from build123d import *

# Parameters (mm, degrees)
SKETCH1_R           = 4
BOSS_EXTRUDE1_DEPTH = 54
SKETCH2_R           = 10
BOSS_EXTRUDE2_DEPTH = 12
SKETCH3_W           = 15
SKETCH3_H           = 30
CUT_EXTRUDE1_DEPTH  = 150
FILLET1_R           = 1


with BuildPart() as part:
    # Sketch1 → Boss-Extrude1 (new body)
    with BuildSketch(Plane.XY):
        with BuildLine():
            Line((0, 75), (0, 20))
            Line((0, 20), (-80, 20))
            ThreePointArc((-80, 20), (-100, 0), (-80, -20))
            Line((-80, -20), (0, -20))
            Line((0, -20), (0, -75))
            Line((0, -75), (15, -75))
            Line((15, -75), (15, 75))
            Line((15, 75), (0, 75))
        make_face()
        with Locations((7.5, 60)):
            Circle(SKETCH1_R, mode=Mode.SUBTRACT)
        with Locations((7.5, -60)):
            Circle(SKETCH1_R, mode=Mode.SUBTRACT)
    extrude(amount=BOSS_EXTRUDE1_DEPTH)

    # Sketch2 → Boss-Extrude2 (add)
    with BuildSketch(Plane(origin=(0, 0, 0), x_dir=(-1, 0, 0), z_dir=(0, 0, -1))):
        with Locations((80, 0)):
            Circle(SKETCH2_R)
    boss_extrude2 = extrude(amount=BOSS_EXTRUDE2_DEPTH)

    # Mirror1: Boss-Extrude2 across plane
    add(boss_extrude2.mirror(Plane.XY.offset(27)))

    # Sketch3 → Cut-Extrude1 (cut)
    with BuildSketch(Plane(origin=(0, 75, 0), x_dir=(1, 0, 0), z_dir=(0, 1, 0))):
        with Locations((7.5, -27)):
            Rectangle(SKETCH3_W, SKETCH3_H)
    extrude(amount=-CUT_EXTRUDE1_DEPTH, mode=Mode.SUBTRACT)

    # Fillet1
    fillet1_edges = [part.edges().sort_by_distance(p)[0] for p in [
        (0, -47.5, 0),
        (-40, -20, 0),
        (-100, 0, 0),
        (0, -47.5, 54),
        (0, 47.5, 54),
        (-40, 20, 54),
        (-100, 0, 54),
        (0, -47.5, 42),
        (0, 47.5, 42),
        (0, -47.5, 12),
        (0, 47.5, 12),
        (-40, 20, 0),
        (-40, -20, 54),
        (0, 47.5, 0),
    ]]
    fillet(fillet1_edges, radius=FILLET1_R)


solid = part.part
Design review of the part built by this model. Coordinates are the model's own, in mm. A direction names the side the tool comes from. Coordinates: 2 decimals unless noted, no trailing zeros. Order: outer loops, then holes, each group sorted by start corner. A loop starts at its lowest first (then second) coordinate and runs counter-clockwise, first axis right, second up. Notation, with made-up numbers: (-18, 15) - (29, 15) arc R22 ccw to (29, 53) - close; hole circle Ø10 at (-1, 11). An arc over 180 degrees is marked (long way). Put each result on its own line as item: value.
1) Take a section at B-B, the plane y = -60. Give the boundary of the cut face in (x, z).
Response values:
outline: (0, 1) arc R1 ccw to (1, 0) - (3.5, 0) - (3.5, 12) - (1, 12) arc R1 ccw to (0, 11) - close; (0, 43) arc R1 ccw to (1, 42) - (3.5, 42) - (3.5, 54) - (1, 54) arc R1 ccw to (0, 53) - close; (11.5, 0) - (15, 0) - (15, 12) - (11.5, 12) - close; (11.5, 42) - (15, 42) - (15, 54) - (11.5, 54) - close
2) The part is to be moulded in two halves that separate along Y. For faces 4 (the face through (8, 75, 48)), 5 (the face through (6.633, -63.905, 47.916)), 6 (the face through (-70, 0, 60)), 7 (the face through (0, -47, 6)), say which applies: released by +Y, released by -Y, zero draft, split by the parting line, or undercut.
Response values:
face 4: released by +Y
face 5: undercut
face 6: split by the parting line
face 7: zero draft
3) Take a section at A-A, the plane x = 7.5. Give the boundary of the cut face in (y, z).
Response values:
outline: (-75, 0) - (-64, 0) - (-64, 12) - (-75, 12) - close; (-75, 42) - (-64, 42) - (-64, 54) - (-75, 54) - close; (-56, 0) - (56, 0) - (56, 12) - (-56, 12) - close; (-56, 42) - (56, 42) - (56, 54) - (-56, 54) - close; (64, 0) - (75, 0) - (75, 12) - (64, 12) - close; (64, 42) - (75, 42) - (75, 54) - (64, 54) - close
4) Take a section at D-D, the plane y = 45.5. Give the boundary of the cut face in (x, z), and give its area (3 significant figures).
Response values:
outline: (0, 1) arc R1 ccw to (1, 0) - (15, 0) - (15, 12) - (1, 12) arc R1 ccw to (0, 11) - close; (0, 43) arc R1 ccw to (1, 42) - (15, 42) - (15, 54) - (1, 54) arc R1 ccw to (0, 53) - close
area: 359 mm²
5) Wall thickness on L1, parallel to Y at x = 7.5, z = 48.5; L2, parallel to Z at x = 9.5, y = -36.5; L3, parallel to X at y = 60, z = 48.75: over which ranges is each line inside the solid? List them lowest first. Write a range as from..to.
Response values:
L1: y = -75..-64, -56..56, 64..75
L2: z = 0..12, 42..54
L3: x = 0..3.5, 11.5..15
6) Insertion check: P1, Ø6, axis at x = -18.5, z = 12, coming from the -Y side; P2, Ø10, axis at y = -16, z = 3.5, coming from the -X side; P3, Ø9, axis at x = 7.5, y = 60, coming from the +Z side. Each pin has a flat end and moves straight along its axis. Give the tip position at first contact, or say it passes through.
Response values:
P1: stops at y = -20
P2: stops at x = -96.7
P3: stops at z = 54
7) Take a section at C-C, the plane z = 4. Give the boundary of the cut face in (x, y).
Response values:
outline: (-80, -20) - (0, -20) - (0, -75) - (15, -75) - (15, 75) - (0, 75) - (0, 20) - (-80, 20) arc R20 ccw to start; hole circle Ø8 at (7.5, -60); hole circle Ø8 at (7.5, 60)
8) Tool access review of faces 1 (the face through (7, 1, 42)), 2 (the face through (-70, 0, -6)), 3 (the face through (0, -47, 48)): name each direction out of +Z, -Z, +X, -X, +Y, -Y from which nothing blocks a thin tool from reaching the whole face with its end or side.
Response values:
face 1: +X, +Y, -Y
face 2: -Z
face 3: +Z, -Z, -X, -Y
